The figure shows three views and two pictorial views of one solid part (mm, origin at its lowest corner). Answer the questions. Coordinates: 2 decimals unless noted, no trailing zeros. Write each loop counter-clockwise with the first axis right and the second up, starting at its lowest first coordinate (ties: lowest second). Pieces come first, ordered by that corner, then holes.
Item 1: Section B-B (y = 50.8) is taken. Give the vertices of the cut face in (x, z), then the cut area to 3 significant figures.
Item 2: Section A-A (z = 95.25) is taken. Give the vertices of the cut face in (x, y), then the cut area to 3 significant figures.
Item 3: Section C-C (x = 2.25) is taken. Give the vertices of the cut face in (y, z).
Item 4: Straight lines are drawn through the part: probe 1 along Y at (x, z) = (2, 95.25); probe 2 along Y at (x, z) = (3, 27); probe 3 along Z at (x, y) = (5.25, 53.5). For each, find the intervals that lie inside material, in ascending order.
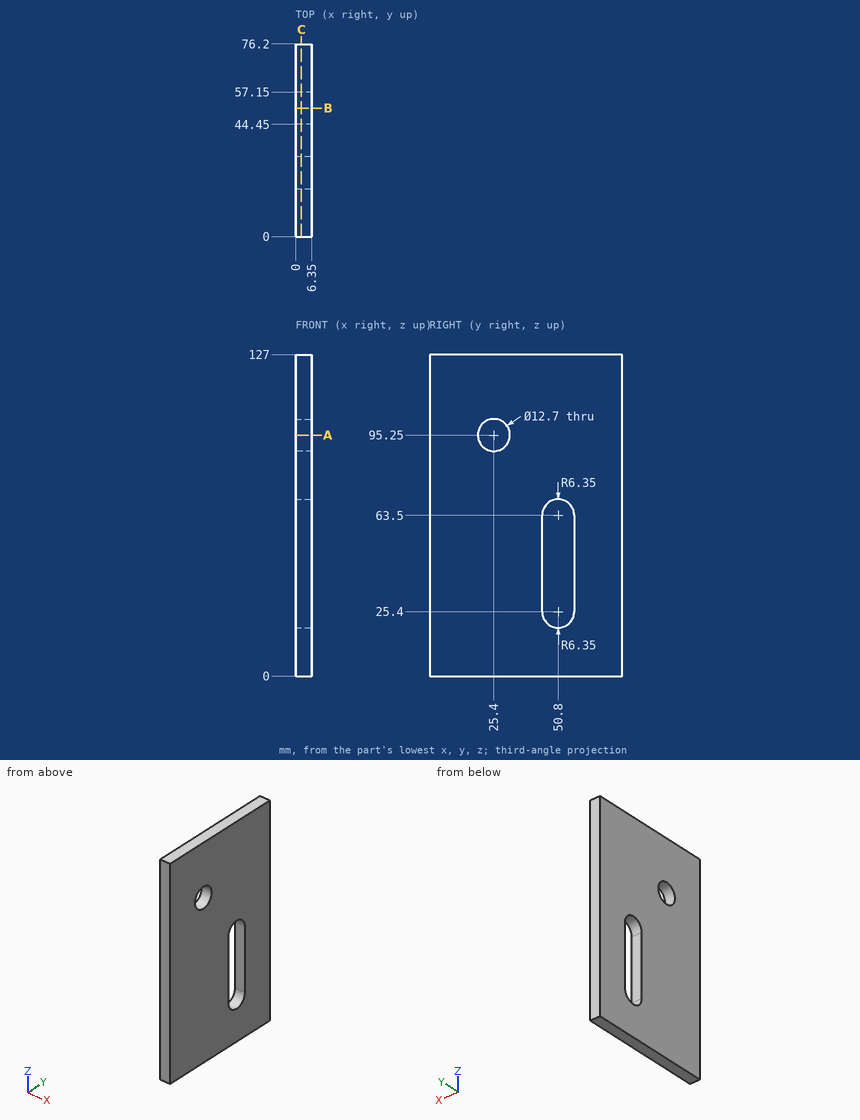
Established:
1. outline: (0, 0) - (6.35, 0) - (6.35, 19.05) - (0, 19.05) - close; (0, 69.85) - (6.35, 69.85) - (6.35, 127) - (0, 127) - close
1. area: 484 mm2
2. outline: (0, 0) - (6.35, 0) - (6.35, 19.05) - (0, 19.05) - close; (0, 31.75) - (6.35, 31.75) - (6.35, 76.2) - (0, 76.2) - close
2. area: 403 mm2
3. outline: (0, 0) - (76.2, 0) - (76.2, 127) - (0, 127) - close; hole circle Ø12.7 at (25.4, 95.25); hole (44.45, 25.4) arc R6.35 ccw to (57.15, 25.4) - (57.15, 63.5) arc R6.35 ccw to (44.45, 63.5) - close
4. probe 1: y = 0 to 19.05, 31.75 to 76.2
4. probe 2: y = 0 to 44.45, 57.15 to 76.2
4. probe 3: z = 0 to 19.65, 69.25 to 127
